from build123d import *

# Parameters (mm, degrees)
SKETCH_W             = 20.859867
SKETCH_H             = 40.764332
PAD_DEPTH            = 6
PAD001_DEPTH         = 1
SKETCH003_R          = 10.454419
PAD002_DEPTH         = 10
SKETCH004_R          = 6.834621
POCKET_DEPTH         = 21.067877
SKETCH005_W          = 8.397711
SKETCH005_H          = 64.60706
POCKET001_DEPTH      = 19.11099
POCKET001_DEPTH_BACK = -1.799848
SKETCH006_R          = 9.297528
PAD003_DEPTH         = 10
SKETCH007_R          = 3.983177
POCKET002_DEPTH      = 11.799848
SKETCH008_W          = 19.389837
SKETCH008_H          = 9.84828
PAD004_DEPTH         = 25
FILLET_R             = 9
SKETCH009_R          = 4.818609
POCKET003_DEPTH      = 15


with BuildPart() as part:
    # Sketch → Pad (new body)
    with BuildSketch(Plane.XY):
        with Locations((-0.636944, -0.955416)):
            Rectangle(SKETCH_W, SKETCH_H)
    extrude(amount=PAD_DEPTH)

    # Sketch002 (on Face2 of Pad) → Pad001 (join, symmetric)
    with BuildSketch(Plane(origin=(-0.20701, 0, -0.1), x_dir=(0, 1, 0), z_dir=(1, 0, 0))):
        Polygon((-21.297264, 17.580976), (-21.297264, 6.008283), (19.375914, 6.008283), align=None)
    extrude(amount=PAD001_DEPTH, both=True)

    # Sketch003 → Pad002 (join, symmetric)
    with BuildSketch(Plane.YZ):
        with Locations((-27.036768, 8.655571)):
            Circle(SKETCH003_R)
    extrude(amount=PAD002_DEPTH, both=True)

    # Sketch004 (on Face13 of Pad002) → Pocket (cut, through all)
    with BuildSketch(Plane.YZ.offset(10)):
        with Locations((-26.973387, 8.428857)):
            Circle(SKETCH004_R)
    extrude(amount=-POCKET_DEPTH, mode=Mode.SUBTRACT)

    # Sketch005 (on Face4 of Pocket) → Pocket001 (cut, two sides)
    with BuildSketch(Plane(origin=(0, 0, 0), x_dir=(1, 0, 0), z_dir=(0, 0, -1))) as pocket001_sk:
        with Locations((-13.88562, 8.634939)):
            Rectangle(SKETCH005_W, SKETCH005_H)
    extrude(amount=-POCKET001_DEPTH, mode=Mode.SUBTRACT)
    extrude(pocket001_sk.sketch, amount=-POCKET001_DEPTH_BACK, mode=Mode.SUBTRACT)

    # Sketch006 → Pad003 (join)
    with BuildSketch(Plane.XY):
        with Locations((0, 20.493547)):
            Circle(SKETCH006_R)
    extrude(amount=PAD003_DEPTH)

    # Sketch007 (on Face15 of Pad003) → Pocket002 (cut, through all)
    with BuildSketch(Plane.XY.offset(10)):
        with Locations((0, 20.013571)):
            Circle(SKETCH007_R)
    extrude(amount=-POCKET002_DEPTH, mode=Mode.SUBTRACT)

    # Sketch008 (on Face2 of Pocket002) → Pad004 (join)
    with BuildSketch(Plane(origin=(0, 0, 0), x_dir=(1, 0, 0), z_dir=(0, 0, -1))):
        with Locations((0.104674, 0.286196)):
            Rectangle(SKETCH008_W, SKETCH008_H)
    extrude(amount=PAD004_DEPTH)

    # Fillet
    fillet_edges = [part.edges().sort_by_distance(p)[0] for p in [
        (-9.590244, -0.286196, -25),
        (9.799593, -0.286196, -25),
    ]]
    fillet(fillet_edges, radius=FILLET_R)

    # Sketch009 (on Face1 of Fillet) → Pocket003 (cut)
    with BuildSketch(Plane(origin=(0, 4.637944, 0), x_dir=(-1, 0, 0), z_dir=(0, 1, 0))):
        with Locations((0, -15.724321)):
            Circle(SKETCH009_R)
    extrude(amount=-POCKET003_DEPTH, mode=Mode.SUBTRACT)


solid = part.part
Part model, mm, in its own coordinate system. A direction names the side the tool comes from. Give positions to 0.01 mm unless a question says otherwise; leave off trailing zeros. Order: outer loops, then holes, each group sorted by start corner. A loop starts at its lowest first (then second) coordinate and runs counter-clockwise, first axis right, second up. Notation, with made-up numbers: (87, 8.25) - (142, 8.25) arc R12 ccw to (142, 22.25) - close; hole circle Ø5 at (87.25, 59.5). An arc over 180 degrees is marked (long way). Use a Markdown table: item, result.
1) Two-plate mould, pull along Z, no slides. Class faces 6 (the cylindrical face through (-7.024, -0.355, -22.294)), 7 (the cylindrical face through (0.294, -23.299, 14.192)), 8 (the flat face through (0, 4.638, -10)): +Z half, -Z half, draft (parallel to the pull), parting line (faces both ways), or undercut.
Checked values:
| item | result |
|---|---|
| face 6 | -Z half |
| face 7 | undercut |
| face 8 | draft |
2) Probe L1, parallel to Y at x = 1.75, z = 5; L2, parallel to Z at x = 4, y = 27.5; L3, parallel to Z at x = 0, y = 0.5. List the from-to ranges inside material, lowest first. Write a range as from..to.
Checked values:
| item | result |
|---|---|
| L1 | -36.83..-32.89, -21.06..16.44, 23.59..29.62 |
| L2 | 0..10 |
| L3 | -25..-20.54, -10.91..11.28 |
3) Saw through at A-A on z = 13. List the corners of the cut face in (x, y), plus the area to 3 significant figures.
Checked values:
| item | result |
|---|---|
| outline | (-9.69, -36.55) - (10, -36.55) - (10, -32.05) - (-9.69, -32.05) - close; (-9.69, -21.89) - (10, -21.89) - (10, -17.53) - (0.79, -17.53) - (0.79, -5.55) - (-1.21, -5.55) - (-1.21, -17.53) - (-9.69, -17.53) - close |
| area | 198 mm² |
4) 3-axis set-ups, long thin cutter, end or side, ignore diameter. For faces 1 (the flat face through (10, -31.83, 13.45)), 2 (the flat face through (4, 18.6, 10)), 3 (the flat face through (0, -5.21, -10)), 4 (the flat face through (-0.19, -4.78, 12.78)), 5 (the cylindrical face through (-1.21, 29.71, 6.04)): which of +Z, -Z, +X, -X, +Y, -Y reach the whole face in a straight line?
Checked values:
| item | result |
|---|---|
| face 1 | +Z, -Z, +X, +Y, -Y |
| face 2 | +Z, +X, -X, +Y |
| face 3 | -Z, +X, -X |
| face 4 | +Z, +X, -X |
| face 5 | +Z |
5) Saw through at D-D on x = 6.5. List the corners of the cut face in (y, z), plus the area to 3 significant figures.
Checked values:
| item | result |
|---|---|
| outline | (-21.17, 0) - (-5.21, 0) - (-5.21, -22.96) - (4.64, -22.96) - (4.64, 0) - (27.14, 0) - (27.14, 10) - (13.85, 10) - (13.85, 6) - (-16.93, 6) arc R10.45 ccw (long way) to start; hole circle Ø13.67 at (-26.97, 8.43) |
| area | 750 mm² |
6) Flat gauge pins, fed straight in: P1, Ø9, axis at x = 0, y = 20.01, coming from the +Z side; P2, Ø4, axis at x = -7.5, y = 2.5, coming from the -Z side; P3, Ø9, axis at y = -6, z = 14, coming from the -X side; P4, Ø8, axis at y = -26.97, z = 8.43, coming from the -X side. Where does each tip first touch, or does it go through?
Checked values:
| item | result |
|---|---|
| P1 | z = 10 |
| P2 | z = -23.54 |
| P3 | x = -1.21 |
| P4 | through |
7) Saw through at B-B on x = -2. List the corners of the cut face in (y, z).
Checked values:
| item | result |
|---|---|
| outline | (-21.17, 0) - (-5.21, 0) - (-5.21, -11.34) - (4.64, -11.34) - (4.64, 0) - (16.57, 0) - (16.57, 10) - (11.41, 10) - (11.41, 6) - (-16.93, 6) arc R10.45 ccw (long way) to start; (-5.21, -24.89) - (4.64, -24.89) - (4.64, -20.11) - (-5.21, -20.11) - close; (23.46, 0) - (29.57, 0) - (29.57, 10) - (23.46, 10) - close; hole circle Ø13.67 at (-26.97, 8.43) |
8) Saw through at C-C on y = -26.5. List the corners of the cut face in (x, z), plus the area to 3 significant figures.
Checked values:
| item | result |
|---|---|
| outline | (-9.69, -1.79) - (10, -1.79) - (10, 1.61) - (-9.69, 1.61) - close; (-9.69, 15.25) - (10, 15.25) - (10, 19.1) - (-9.69, 19.1) - close |
| area | 143 mm² |
